Could you check a few things on this model? Use its own coordinates, in mm. A direction names the side the tool comes from. Round coordinates to 2 decimals unless told otherwise and drop trailing zeros. Loops run counter-clockwise (first coordinate to the right, second up) from the corner with the lowest first, then second, coordinate; pieces in that order, holes last. Notation, with made-up numbers: (28, 61) -> (54, 61) arc R19 ccw to (54, 80) -> close; hole circle Ø9 at (-14, 58). An arc over 180 degrees is marked (long way). One line per item, written item: value.
```python
from build123d import *

# Parameters (mm, degrees)
BOSS_EXTRU_1_DEPTH      = 10
ESQUISSE2_R             = 1.5
ESQUISSE2_R_2           = 2.3
ENL_V_MAT_EXTRU_1_DEPTH = 54.203009486


with BuildPart() as part:
    # Esquisse1 → Boss.-Extru.1 (new body)
    with BuildSketch(Plane.XY):
        with BuildLine():
            Line((-17.240327137, -13.100674555), (-17.240327137, -2.100674555))
            ThreePointArc((-17.240327137, -2.100674555), (-16.947433918, -1.393567773), (-16.240327137, -1.100674555))
            ThreePointArc((-16.240327137, -1.100674555), (-15.533220355, -0.807781336), (-15.240327137, -0.100674555))
            Line((-15.240327137, -0.100674555), (-15.240327137, 15.899325445))
            ThreePointArc((-15.240327137, 15.899325445), (-14.947433918, 16.606432227), (-14.240327137, 16.899325445))
            Line((-14.240327137, 16.899325445), (-8.740327137, 16.899325445))
            ThreePointArc((-8.740327137, 16.899325445), (-8.033220355, 17.192218664), (-7.740327137, 17.899325445))
            Line((-7.740327137, 17.899325445), (-7.740327137, 36.899325445))
            Line((-7.740327137, 36.899325445), (-4.740327137, 36.899325445))
            Line((-4.740327137, 36.899325445), (-4.740327137, 15.899325445))
            ThreePointArc((-4.740327137, 15.899325445), (-4.447433918, 15.192218664), (-3.740327137, 14.899325445))
            Line((-3.740327137, 14.899325445), (6.259672863, 14.899325445))
            ThreePointArc((6.259672863, 14.899325445), (6.966779645, 15.192218664), (7.259672863, 15.899325445))
            Line((7.259672863, 15.899325445), (7.259672863, 36.899325445))
            Line((7.259672863, 36.899325445), (10.259672863, 36.899325445))
            Line((10.259672863, 36.899325445), (10.259672863, 17.899325445))
            ThreePointArc((10.259672863, 17.899325445), (10.552566082, 17.192218664), (11.259672863, 16.899325445))
            Line((11.259672863, 16.899325445), (16.759672863, 16.899325445))
            ThreePointArc((16.759672863, 16.899325445), (17.466779645, 16.606432227), (17.759672863, 15.899325445))
            Line((17.759672863, 15.899325445), (17.759672863, -0.100674555))
            ThreePointArc((17.759672863, -0.100674555), (18.052566082, -0.807781336), (18.759672863, -1.100674555))
            ThreePointArc((18.759672863, -1.100674555), (19.466779645, -1.393567773), (19.759672863, -2.100674555))
            Line((19.759672863, -2.100674555), (19.759672863, -13.100674555))
            Line((19.759672863, -13.100674555), (14.759672863, -13.100674555))
            Line((14.759672863, -13.100674555), (14.759672863, 10.899325445))
            ThreePointArc((14.759672863, 10.899325445), (14.466779645, 11.606432227), (13.759672863, 11.899325445))
            Line((13.759672863, 11.899325445), (-11.240327137, 11.899325445))
            ThreePointArc((-11.240327137, 11.899325445), (-11.947433918, 11.606432227), (-12.240327137, 10.899325445))
            Line((-12.240327137, 10.899325445), (-12.240327137, -13.100674555))
            Line((-12.240327137, -13.100674555), (-17.240327137, -13.100674555))
        make_face()
    extrude(amount=BOSS_EXTRU_1_DEPTH)

    # Esquisse2 → Enlèv. mat.-Extru.1 (cut, through all)
    with BuildSketch(Plane.ZY.offset(17.240327137)):
        with BuildLine():
            Line((0, 36.899325445), (0, 31.899325445))
            ThreePointArc((0, 31.899325445), (1.464466094, 35.434859351), (5, 36.899325445))
            Line((5, 36.899325445), (0, 36.899325445))
        make_face()
        with BuildLine():
            Line((10, 36.899325445), (5, 36.899325445))
            ThreePointArc((5, 36.899325445), (8.535533906, 35.434859351), (10, 31.899325445))
            Line((10, 31.899325445), (10, 36.899325445))
        make_face()
        with BuildLine():
            ThreePointArc((10, -8.100674555), (8.535533906, -11.636208461), (5, -13.100674555))
            Line((5, -13.100674555), (10, -13.100674555))
            Line((10, -13.100674555), (10, -8.100674555))
        make_face()
        with BuildLine():
            ThreePointArc((5, -13.100674555), (1.464466094, -11.636208461), (0, -8.100674555))
            Line((0, -8.100674555), (0, -13.100674555))
            Line((0, -13.100674555), (5, -13.100674555))
        make_face()
        with Locations(Location((5, 31.899325445, 0), (0, 0, 90))):
            Circle(ESQUISSE2_R)
        with Locations((5, -8.100674555)):
            Circle(ESQUISSE2_R_2)
    extrude(amount=-ENL_V_MAT_EXTRU_1_DEPTH, mode=Mode.SUBTRACT)


solid = part.part
```
Item 1: If we section it at A-A on x = -5.5: List the corners of the cut face in (y, z) for me, plus the area to 3 significant figures.
Output:
outline: (11.9, 0) -> (31.9, 0) arc R5 ccw to (31.9, 10) -> (11.9, 10) -> close; hole circle Ø3 at (31.9, 5)
area: 232 mm²
Item 2: If we section it at C-C on z = 5.75: Count the separate pieces of the cut face and the enclosed holes in it, plus the area to 3 significant figures.
Output:
separate pieces: 5
enclosed holes: 0
area: 400 mm²
Item 3: I need wall thicknesses on line 1 (X direction, y = 9.5, z = 1.75); line 2 (X direction, y = 27, z = 6.5); line 3 (Y direction, x = 18.65, z = 5). Which ranges of each line are inside material? Lowest first, please. Write a range as from..to.
Output:
line 1: x = -15.24..-12.24, 14.76..17.76
line 2: x = -7.74..-4.74, 7.26..10.26
line 3: y = -13.1..-10.4, -5.8..-1.09
Item 4: Will these pins go through, and if not, where does the flat tip stop? pin 1 Ø3 at (y, z) = (22.5, 6.5) entering from -X; pin 2 Ø10 at (x, y) = (12.5, 0) entering from +Z; pin 3 Ø3 at (y, z) = (7.5, 4.5) entering from -X; pin 4 Ø2.5 at (x, z) = (12.5, 3) entering from +Y.
Output:
pin 1: stops at x = -7.74
pin 2: stops at z = 10
pin 3: stops at x = -15.24
pin 4: stops at y = 16.9
Item 5: If we mould it in two halves opening along Z, with no side actions, what happens to faces 4 (the face through (-3, 13, 10)), 5 (the face through (8.74, 33.33, 4.55)), 6 (the face through (-17.24, -5, 5))? For each: released by +Z, released by -Z, zero draft, split by the parting line, or undercut.
Output:
face 4: released by +Z
face 5: undercut
face 6: zero draft
Item 6: For faces 1 (the face through (-15.24, 8, 5)), 2 (the face through (14, 16.899, 5)), 3 (the face through (1, 11.899, 5)), which set-ups out of +Z, -Z, +X, -X, +Y, -Y let a thin tool reach every point of the face, with its end or its side?
Output:
face 1: +Z, -Z, -X, +Y
face 2: +Z, -Z, +X, +Y
face 3: +Z, -Z, -Y
